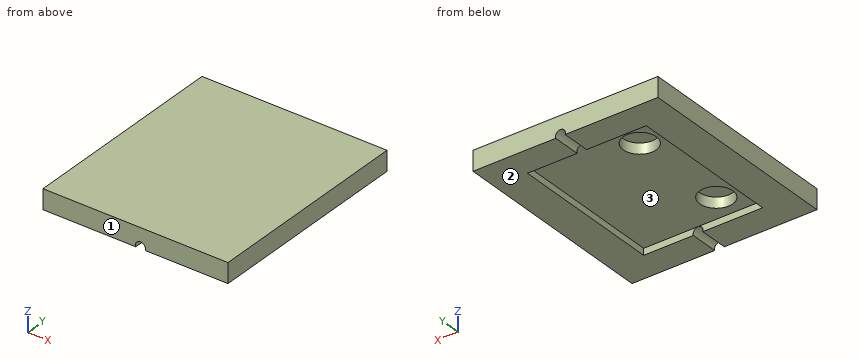
Autodesk Inventor part; units mm, degrees
ref_plane "Work Plane2" through (-6.35, -9.05, 2.6) normal (0, 0, 1) x (1, 0, 0)
ref_plane "YZ Plane" through (0, 0, 0) normal (1, 0, 0) x (0, 1, 0)
ref_plane "XZ Plane" through (0, 0, 0) normal (0, 1, 0) x (-1, 0, 0)
ref_plane "Work Plane1" through (0, 0, 0) normal (0, 0, 1) x (1, 0, 0)
sketch "Sketch1" plane through (0, 0, 0) normal (0, 0, 1) x (1, 0, 0)
  arc A0 (2.9937, -6.1068) -> (2.9937, 6.1788) centre (1.841, 0.036) ccw
  line L0 (2.9937, -6.1068) -> (2.9937, -9.05)
  line L1 (2.9937, -9.05) -> (-5, -9.05)
  arc A1 (-5, -6.35) -> (-5, -9.05) centre (-5, -7.7) ccw
  line L2 (-5, -6.35) -> (-0.5216, -6.35)
  line L3 (-0.5216, -6.35) -> (-0.5216, -5.7502)
  arc A2 (-0.9246, 5.6409) -> (-0.5216, -5.7502) centre (1.841, 0.036) ccw
  line L4 (-0.9246, 5.6409) -> (-0.9246, 6.35)
  line L5 (-0.9246, 6.35) -> (-5, 6.35)
  arc A3 (-5, 9.05) -> (-5, 6.35) centre (-5, 7.7) ccw
  line L6 (-5, 9.05) -> (2.9937, 9.05)
  line L7 (2.9937, 9.05) -> (2.9937, 6.1788)
  line L8 (14, -16) -> (-14, -16)
  line L9 (14, 16) -> (14, -16)
  line L10 (-14, 16) -> (14, 16)
  line L11 (-14, -16) -> (-14, 16)
  point P0 (0, 0)
extrude "Extrusion1" add sketch "Sketch1" along normal blind 3 contours L0 L1 A1 L2 L3 A2 L4 L5 A3 L6 L7 A0 | L8 L11 L10 L9
sketch "Sketch2" plane through (0, 0, 3) normal (0, 0, 1) x (1, 0, 0)
  circle A0 centre (-5, 7.7) radius 1.35
  circle A1 centre (-5, -7.7) radius 1.35
  circle A2 centre (1.841, 0.036) radius 5
  circle A3 centre (1.841, 0.036) radius 5.2
  circle A4 centre (-5, 7.7) radius 1.55
  point P0 (0, 0)
  dimension "d2" = 0.2
  dimension "d3" = 0.2
sketch "Sketch3" plane through (0, 0, 0) normal (0, 0, -1) x (-1, 0, 0)
  circle A0 centre (5, 7.7) radius 2.5
  circle A1 centre (5, -7.7) radius 2.5
  point P0 (0, 0)
extrude "Extrusion2" cut sketch "Sketch3" against normal through all
sketch "Sketch4" plane through (0, 0, 0) normal (0, 0, -1) x (-1, 0, 0)
  line L0 (-14, -16) -> (14, -16)
  line L1 (14, -16) -> (14, 16)
  line L2 (14, 16) -> (-14, 16)
  line L3 (-14, 16) -> (-14, -16)
  line L4 (9, -11.7) -> (9, 11.7)
  line L5 (-9, -11.7) -> (9, -11.7)
  line L6 (-9, 11.7) -> (-9, -11.7)
  line L7 (9, 11.7) -> (-9, 11.7)
  point P0 (0, 0)
extrude "Extrusion3" cut sketch "Sketch4" against normal blind 1 contours L5 L6 L7 L4
sketch "Sketch5" plane through (0, 0, 3) normal (0, 0, 1) x (1, 0, 0)
  circle A0 centre (-5, 7.7) radius 2.5
  circle A1 centre (-5, -7.7) radius 2.5
  point P0 (0, 0)
ref_plane "Work Plane2" through (-6.35, -9.05, 2.6) normal (0, 0, 1) x (1, 0, 0)
extrude "Extrusion4" add sketch "Sketch5" against normal up to surface (0.4 mm away)
sketch "Sketch6" plane through (-14, 16, 0) normal (0, 1, 0) x (1, 0, 0)
  line L0 (23, -1) -> (5, -1)
  line L1 (0, 0) -> (28, 0)
  line L2 (0, 0) -> (0, -3)
  line L3 (28, -3) -> (0, -3)
  line L4 (28, 0) -> (28, -3)
  circle A0 centre (14.7595, -0.2282) radius 0.75
  dimension "d11" = 1.5
extrude "Extrusion5" cut sketch "Sketch6" against normal through all contours A0 L1 | L1 A0
properties part number "00_PDMS_mould_1"
Could you check a few things on this model? Use its own coordinates, in mm. Face numbers are marked on the shaded views. Coordinates: 2 decimals unless noted, no trailing zeros. Order: outer loops, then holes, each group sorted by start corner. A loop starts at its lowest first (then second) coordinate and runs counter-clockwise, first axis right, second up. Notation, with made-up numbers: (-36, -5) -> (-2, -5) arc R8 ccw to (-2, 4) -> close; hole circle Ø4 at (36, 67.5). An arc over 180 degrees is marked (long way). One line per item, written item: value. Start each with the question number.
1) We'd pull the mould along Y, two halves only. Please class the marked faces 1, 2 and 3: +Y half, -Y half, draft (parallel to the pull), parting line (faces both ways), or undercut.
2) Imagine slicing it at A-A on z = 0.6. List the corners of the cut face in (x, y) for me.
3) I'm going to push flat-ended pins straight in: pin 1 (10 mm diameter, centred on x = -10, y = -12.5, fed in from -Z); pin 2 (3 mm diameter, centred on x = -5, y = -7.7, fed in from -Z); pin 3 (14.5 mm diameter, centred on x = 0, y = 0, fed in from -Z). Where does each tip first touch, or does it pass through?
4) Imagine slicing it at C-C on x = -1.75. List the corners of the cut face in (y, z) for me.
5) Imagine slicing it at B-B on y = 1.5. List the corners of the cut face in (x, z) for me, plus the area to 3 significant figures.
6) If I drill on L1, parallel to Y at x = -5, z = 2.35; L2, parallel to X at y = -8, z = 0.25; L3, parallel to Z at x = -4.5, y = 1, over which ranges is the centre line in solid material (lowest first)? Write a range as [from, to].
7) Imagine slicing it at D-D on y = 7.7. List the corners of the cut face in (x, z) for me, plus the area to 3 significant figures.
Answer list:
1. face 1: -Y half
1. face 2: draft
1. face 3: undercut
2. outline: (-14, -16) -> (0.11, -16) -> (0.11, -11.7) -> (-9, -11.7) -> (-9, 11.7) -> (0.11, 11.7) -> (0.11, 16) -> (-14, 16) -> close; (1.41, -16) -> (14, -16) -> (14, 16) -> (1.41, 16) -> (1.41, 11.7) -> (9, 11.7) -> (9, -11.7) -> (1.41, -11.7) -> close
3. pin 1: stops at z = 0
3. pin 2: stops at z = 2.6
3. pin 3: stops at z = 1
4. outline: (-16, 0) -> (-11.7, 0) -> (-11.7, 1) -> (11.7, 1) -> (11.7, 0) -> (16, 0) -> (16, 3) -> (-16, 3) -> close
5. outline: (-14, 0) -> (-9, 0) -> (-9, 1) -> (9, 1) -> (9, 0) -> (14, 0) -> (14, 3) -> (-14, 3) -> close
5. area: 66.0 mm2
6. L1: y = [-16, -10.2], [-5.2, 5.2], [10.2, 16]
6. L2: x = [-14, -9], [9, 14]
6. L3: z = [1, 3]
7. outline: (-14, 0) -> (-9, 0) -> (-9, 1) -> (-7.5, 1) -> (-7.5, 2.6) -> (-2.5, 2.6) -> (-2.5, 1) -> (9, 1) -> (9, 0) -> (14, 0) -> (14, 3) -> (-14, 3) -> close
7. area: 58.0 mm2
